Here's how the part is built. I have some questions about the finished solid (model axes, mm). Face numbers are marked on the shaded views. A direction names the side the tool comes from. Give positions to 0.01 mm unless a question says otherwise; leave off trailing zeros. Loops run counter-clockwise (first coordinate to the right, second up) from the corner with the lowest first, then second, coordinate; pieces in that order, holes last. Notation, with made-up numbers: (12, 35.25) - (19, 35.25) arc R36 ccw to (19, 72.25) - close; hole circle Ø11 at (41, 32.5). An arc over 180 degrees is marked (long way). Use one line per item in the form item = value.
from build123d import *

# Parameters (mm, degrees)
F0_R      = 7.7
F1_DEPTH  = 4
F2_R      = 10
F2_R_2    = 7.7
F3_DEPTH  = 1
F4_R      = 10
F4_R_2    = 7.7
F5_DEPTH  = 1
F6_R      = 5.5
F7_DEPTH  = 6
F9_D      = 4
F10_R     = 1.5
F11_DEPTH = 25


with BuildPart() as f1:
    # F0 (on Top) → F1 (new body, symmetric)
    with BuildSketch(Plane.XY):
        Circle(F0_R)
    extrude(amount=F1_DEPTH, both=True)

    # F2 (on face) → F3 (join)
    with BuildSketch(Plane.XY.offset(4)):
        Circle(F2_R)
        Circle(F2_R_2, mode=Mode.SUBTRACT)
        Circle(F2_R_2)
    extrude(amount=F3_DEPTH)

    # F4 (on face) → F5 (join)
    with BuildSketch(Plane(origin=(0, 0, -4), x_dir=(1, 0, 0), z_dir=(0, 0, -1))):
        Circle(F4_R)
        Circle(F4_R_2, mode=Mode.SUBTRACT)
        Circle(F4_R_2)
    extrude(amount=F5_DEPTH)

    # F6 (on face) → F7 (join)
    with BuildSketch(Plane.XY.offset(5)):
        Circle(F6_R)
    extrude(amount=F7_DEPTH)

    # F9 (through all)
    with Locations(Plane.XY.offset(11)):
        with Locations((0, 0)):
            Hole(F9_D / 2)

    # F10 (on Front) → F11 (cut)
    with BuildSketch(Plane.XZ):
        with Locations((0, 8)):
            Circle(F10_R)
    extrude(amount=F11_DEPTH, mode=Mode.SUBTRACT)


solid = f1.part
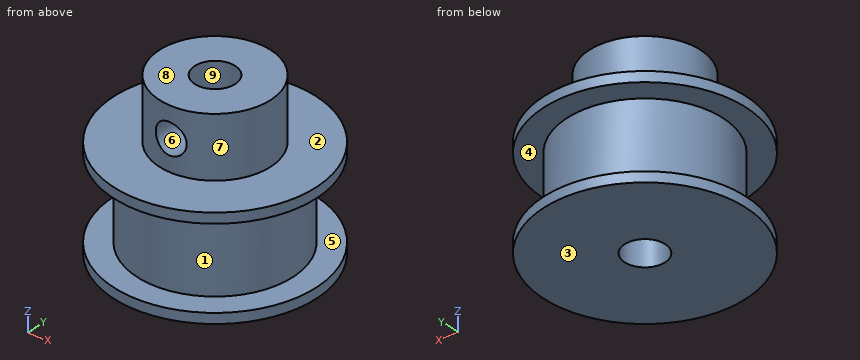
(1) If we section it at C-C (z = 1): List the corners of the cut face in (x, y) for me, plus the area to 3 significant figures.
Geometry says:
outline = circle Ø15.4 at (0, 0); hole circle Ø4 at (0, 0)
area = 174 mm²
(2) If we section it at B-B (x = 0): List the corners of the cut face in (y, z) for me.
Geometry says:
outline = (-10, -5) - (-2, -5) - (-2, 6.5) - (-5.5, 6.5) - (-5.5, 5) - (-10, 5) - (-10, 4) - (-7.7, 4) - (-7.7, -4) - (-10, -4) - close; (-5.5, 9.5) - (-2, 9.5) - (-2, 11) - (-5.5, 11) - close; (2, -5) - (10, -5) - (10, -4) - (7.7, -4) - (7.7, 4) - (10, 4) - (10, 5) - (5.5, 5) - (5.5, 11) - (2, 11) - close
(3) Thinking about a two-plate mould opening in Z: for the marked faces 1, 2, 3 and 4, which applies, pulls with the +Z half, pulls with the -Z half, needs draft (parallel to the pull), parting line crosses it, or undercut?
Geometry says:
face_1 = undercut
face_2 = pulls with the +Z half
face_3 = pulls with the -Z half
face_4 = undercut
(4) For the marked faces 5, 6, 7, 8 and 9, which set-ups out of +Z, -Z, +X, -X, +Y, -Y let a thin tool reach every point of the face, with its end or its side?
Geometry says:
face_5 = none
face_6 = -Y
face_7 = +Z
face_8 = +Z, +X, -X, +Y, -Y
face_9 = +Z, -Z
(5) If we section it at A-A (y = 0): List the corners of the cut face in (x, z) for me, plus the area to 3 significant figures.
Geometry says:
outline = (-10, -5) - (-2, -5) - (-2, 11) - (-5.5, 11) - (-5.5, 5) - (-10, 5) - (-10, 4) - (-7.7, 4) - (-7.7, -4) - (-10, -4) - close; (2, -5) - (10, -5) - (10, -4) - (7.7, -4) - (7.7, 4) - (10, 4) - (10, 5) - (5.5, 5) - (5.5, 11) - (2, 11) - close
area = 165 mm²
(6) For P1, Ø5, axis at x = 0, z = 8, coming from the -Y side; P2, Ø2, axis at x = 7.5, z = 7.5, coming from the -Y side; P3, Ø2, axis at x = 7.5, y = -7, coming from the +Z side; P4, Ø4, axis at y = 5.5, z = 3, coming from the +X side, each with a flat end and sliding along its axis, tell me the tip position at first contact or that it passes through.
Geometry says:
P1 = -5.5
P2 = through
P3 = 5
P4 = 9.26
(7) If I drill on probe 1 along Z at (x, y) = (6.5, 6.5); probe 2 along Y at (x, z) = (0, 1.25); probe 3 along Z at (x, y) = (0, -3.5), over which ranges is the centre line in solid material (lowest first)?
Geometry says:
probe_1 = -5 to -4, 4 to 5
probe_2 = -7.7 to -2, 2 to 7.7
probe_3 = -5 to 6.5, 9.5 to 11
(8) If we section it at D-D (y = -4.75): List the corners of the cut face in (x, z) for me.
Geometry says:
outline = (-8.8, -5) - (8.8, -5) - (8.8, -4) - (6.06, -4) - (6.06, 4) - (8.8, 4) - (8.8, 5) - (2.77, 5) - (2.77, 11) - (-2.77, 11) - (-2.77, 5) - (-8.8, 5) - (-8.8, 4) - (-6.06, 4) - (-6.06, -4) - (-8.8, -4) - close; hole circle Ø3 at (0, 8)
